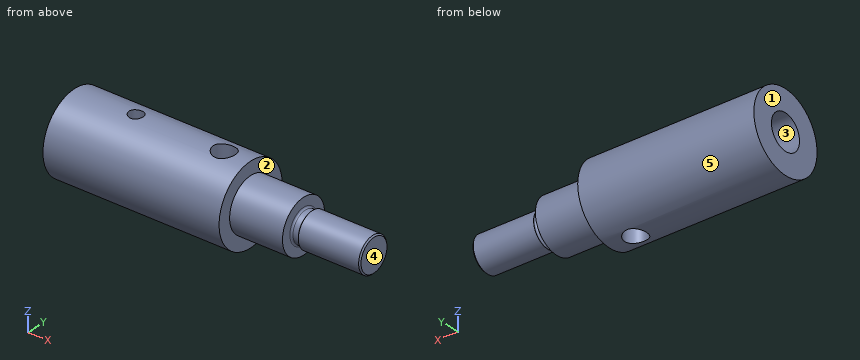
```python
from build123d import *

# Parameters (mm, degrees)
FASE1_SIZE                           = 0.15
SKIZZE2_W                            = 1
SKIZZE2_H                            = 0.5
VERRUNDUNG1_R                        = 0.2
SKIZZE5_W                            = 0.8
SKIZZE5_H                            = 4.5
SKIZZE7_R                            = 1.25
SCHNITT_LINEAR_AUSTRAGEN2_DEPTH      = 5.50000011
SCHNITT_LINEAR_AUSTRAGEN2_DEPTH_BACK = 5.5000001


with BuildPart() as part:
    # Skizze1 → Rotation1 (revolve)
    with BuildSketch(Plane.XY):
        Polygon((0, 4.5), (0, 2), (14, 2), (15.201721238, 0), (34, 0), (34, 2), (26, 2), (26, 3), (20, 3), (20, 4.5), align=None)
    revolve(axis=Axis((0, 0, 0), (1, 0, 0)))

    # Fase1
    fase1_edges = [part.edges().sort_by_distance(p)[0] for p in [
        (34, -2, 0),
    ]]
    chamfer(fase1_edges, length=FASE1_SIZE)

    # Skizze2 → Schnitt-Rotation1 (revolve, cut)
    with BuildSketch(Plane.XY):
        with Locations((26.5, 2)):
            Rectangle(SKIZZE2_W, SKIZZE2_H)
    revolve(axis=Axis((0, 0, 0), (1, 0, 0)), mode=Mode.SUBTRACT)

    # Verrundung1
    verrundung1_edges = [part.edges().sort_by_distance(p)[0] for p in [
        (27, -1.75, 0),
        (26, -1.75, 0),
    ]]
    fillet(verrundung1_edges, radius=VERRUNDUNG1_R)

    # Skizze5 → M2 Gewindebohrung1 (revolve, cut)
    with BuildSketch(Plane.YZ.offset(7)):
        with Locations((0.4, 2.25)):
            Rectangle(SKIZZE5_W, SKIZZE5_H)
    revolve(axis=Axis((7, 0, -6.35), (0, 0, 1)), mode=Mode.SUBTRACT)

    # Skizze7 → Schnitt-Linear austragen2 (cut, two sides)
    with BuildSketch(Plane.XY) as schnitt_linear_austragen2_sk:
        with Locations((17, 0)):
            Circle(SKIZZE7_R)
    extrude(amount=SCHNITT_LINEAR_AUSTRAGEN2_DEPTH, mode=Mode.SUBTRACT)
    extrude(schnitt_linear_austragen2_sk.sketch, amount=-SCHNITT_LINEAR_AUSTRAGEN2_DEPTH_BACK, mode=Mode.SUBTRACT)


solid = part.part
```
The model under review builds one solid part; all positions refer to its coordinate system, in mm. Face numbers are marked on the shaded views. A direction names the side the tool comes from. Give positions to 0.01 mm unless a question says otherwise; leave off trailing zeros. Write each loop counter-clockwise with the first axis right and the second up, starting at its lowest first coordinate (ties: lowest second). Pieces come first, ordered by that corner, then holes. Notation, with made-up numbers: (15, 13.5) -> (49, 13.5) arc R25 cw to (49, 28.5) -> close; hole circle Ø2 at (19.25, 32.25). An arc over 180 degrees is marked (long way). Answer in a Markdown table with one row per item.
1) Add section D-D on x = 17. State the section outline as (y, z) points, plus the area to 3 significant figures.
Worked answers:
| item | result |
|---|---|
| outline | (-1.25, -4.32) -> (-1.25, 4.32) arc R4.5 ccw to start; (1.25, -4.32) arc R4.5 ccw to (1.25, 4.32) -> close |
| area | 41.4 mm² |
2) For L1, parallel to X at y = 0, z = -1.8; L2, parallel to X at y = 0, z = -2.35; L3, parallel to X at y = -1, z = -1.25, list the stretches that pass through material, from the lowest coordinate up. Write a range as [from, to].
Worked answers:
| item | result |
|---|---|
| L1 | [14.12, 15.75], [18.25, 26.07], [26.93, 34] |
| L2 | [0, 15.75], [18.25, 26] |
| L3 | [14.24, 16.25], [17.75, 34] |
3) Add section A-A on z = 3.75. State the section outline as (x, y) points.
Worked answers:
| item | result |
|---|---|
| outline | (0, -2.49) -> (20, -2.49) -> (20, 2.49) -> (0, 2.49) -> close; hole circle Ø1.6 at (7, 0); hole circle Ø2.5 at (17, 0) |
4) Tool access review of the marked faces 1 and 2: name each direction out of +Z, -Z, +X, -X, +Y, -Y from which nothing blocks a thin tool from reaching the whole face with its end or side.
Worked answers:
| item | result |
|---|---|
| face 1 | +Z, -Z, -X, +Y, -Y |
| face 2 | +X |
5) Mouldability with a two-part tool opening along Z and no side actions: class the marked faces 3, 4 and 5 as +Z half, -Z half, draft (parallel to the pull), parting line (faces both ways), or undercut.
Worked answers:
| item | result |
|---|---|
| face 3 | undercut |
| face 4 | draft |
| face 5 | parting line |
6) Clearance check with flat-ended pins moving along their axes: P1, Ø2, axis at y = 0, z = -0.5, coming from the -X side; P2, Ø4, axis at x = 18, y = -3, coming from the -Z side; P3, Ø1.3, axis at x = 7, y = 0, coming from the +Z side; P4, Ø1.5, axis at y = -1.5, z = 1.5, coming from the -X side. State where each tip first meets the part, or that it passes through.
Worked answers:
| item | result |
|---|---|
| P1 | x = 14.3 |
| P2 | z = -4.39 |
| P3 | z = -1.89 |
| P4 | x = 0 |
7) Add section C-C on y = -3.5. State the section outline as (x, z) points, plus the area to 3 significant figures.
Worked answers:
| item | result |
|---|---|
| outline | (0, -2.83) -> (20, -2.83) -> (20, 2.83) -> (0, 2.83) -> close |
| area | 113 mm² |
8) Add section B-B on x = 3.5. State the section outline as (y, z) points, plus the area to 3 significant figures.
Worked answers:
| item | result |
|---|---|
| outline | circle Ø9 at (0, 0); hole circle Ø4 at (0, 0) |
| area | 51.1 mm² |
